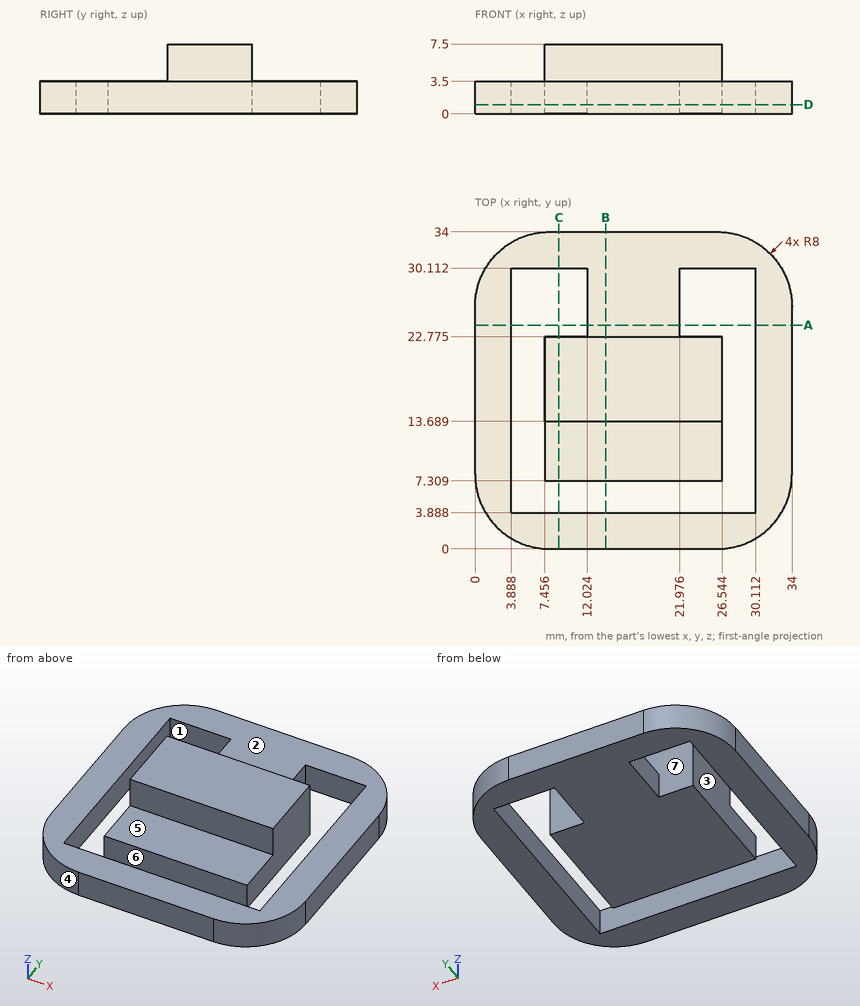
Study the drawing (mm; zero at the part's minimum x, y, z) and answer. A direction names the side the tool comes from. Coordinates: 2 decimals unless noted, no trailing zeros. Write each loop counter-clockwise with the first axis right and the second up, starting at its lowest first coordinate (ties: lowest second). Pieces come first, ordered by that corner, then holes. Notation, with made-up numbers: (81, -29) - (114, -29) arc R20 ccw to (114, -23) - close; hole circle Ø9 at (70.25, 86.5). An arc over 180 degrees is marked (long way). Answer as a JSON object with one key per item and string values.
Q1. For a pull along X with two mould halves and no side action, classify the marked faces 1, 2, 3 and 4 as pulls with the +X half, pulls with the -X half, needs draft (parallel to the pull), parting line crosses it, or undercut.
Results list:
{"face 1": "undercut", "face 2": "needs draft", "face 3": "undercut", "face 4": "pulls with the -X half"}
Q2. Find section A-A (y = 24). Write down the section's boundary in (x, z).
Results list:
{"outline": "(0, 0) - (3.89, 0) - (3.89, 3.5) - (0, 3.5) - close; (12.02, 0) - (21.98, 0) - (21.98, 3.5) - (12.02, 3.5) - close; (30.11, 0) - (34, 0) - (34, 3.5) - (30.11, 3.5) - close"}
Q3. Find section D-D (z = 1). Write down the section's boundary in (x, y) (1 decimal).
Results list:
{"outline": "(0, 8) arc R8 ccw to (8, 0) - (26, 0) arc R8 ccw to (34, 8) - (34, 26) arc R8 ccw to (26, 34) - (8, 34) arc R8 ccw to (0, 26) - close; hole (3.9, 3.9) - (30.1, 3.9) - (30.1, 30.1) - (22, 30.1) - (22, 22.8) - (26.5, 22.8) - (26.5, 7.3) - (7.5, 7.3) - (7.5, 22.8) - (12, 22.8) - (12, 30.1) - (3.9, 30.1) - close"}
Q4. Given pin 1 Ø2 at (y, z) = (6.5, 4) entering from -X (1 decimal); pin 2 Ø3 at (x, y) = (17.5, 9) entering from +Z; pin 3 Ø1.5 at (y, z) = (20.5, 5) entering from -X, each flat-ended and moving along its own axis, determine where each tip first touches the part or whether it passes through.
Results list:
{"pin 1": "stops at x = 0", "pin 2": "stops at z = 3.5", "pin 3": "stops at x = 7.46"}
Q5. Find section C-C (x = 9). Write down the section's boundary in (y, z) (1 decimal), plus the area to 3 significant figures.
Results list:
{"outline": "(0, 0) - (3.9, 0) - (3.9, 3.5) - (0, 3.5) - close; (7.3, 0) - (22.8, 0) - (22.8, 7.5) - (13.7, 7.5) - (13.7, 3.5) - (7.3, 3.5) - close; (30.1, 0) - (34, 0) - (34, 3.5) - (30.1, 3.5) - close", "area": "118 mm^2"}
Q6. Consider L1, parallel to X at y = 20, z = 3.25 (1 decimal); L2, parallel to X at y = 23, z = 3; L3, parallel to Y at x = 25, z = 2 (1 decimal). Determine where each line is inside the solid, lowest interval first. Write a range as from..to.
Results list:
{"L1": "x = 0..3.9, 7.5..26.5, 30.1..34", "L2": "x = 0..3.89, 12.02..21.98, 30.11..34", "L3": "y = 0..3.9, 7.3..22.8, 30.1..34"}
Q7. Which of the six approach directions +Z, -Z, +X, -X, +Y, -Y give full straight-line access (tool end or side, diameter ignored) to the marked faces 5, 6 and 7?
Results list:
{"face 5": "+Z, +X, -X, -Y", "face 6": "+Z, -Z", "face 7": "+Z"}
Q8. Find section B-B (x = 14). Write down the section's boundary in (y, z) (1 decimal), plus the area to 3 significant figures.
Results list:
{"outline": "(0, 0) - (3.9, 0) - (3.9, 3.5) - (0, 3.5) - close; (7.3, 0) - (34, 0) - (34, 3.5) - (22.8, 3.5) - (22.8, 7.5) - (13.7, 7.5) - (13.7, 3.5) - (7.3, 3.5) - close", "area": "143 mm^2"}
